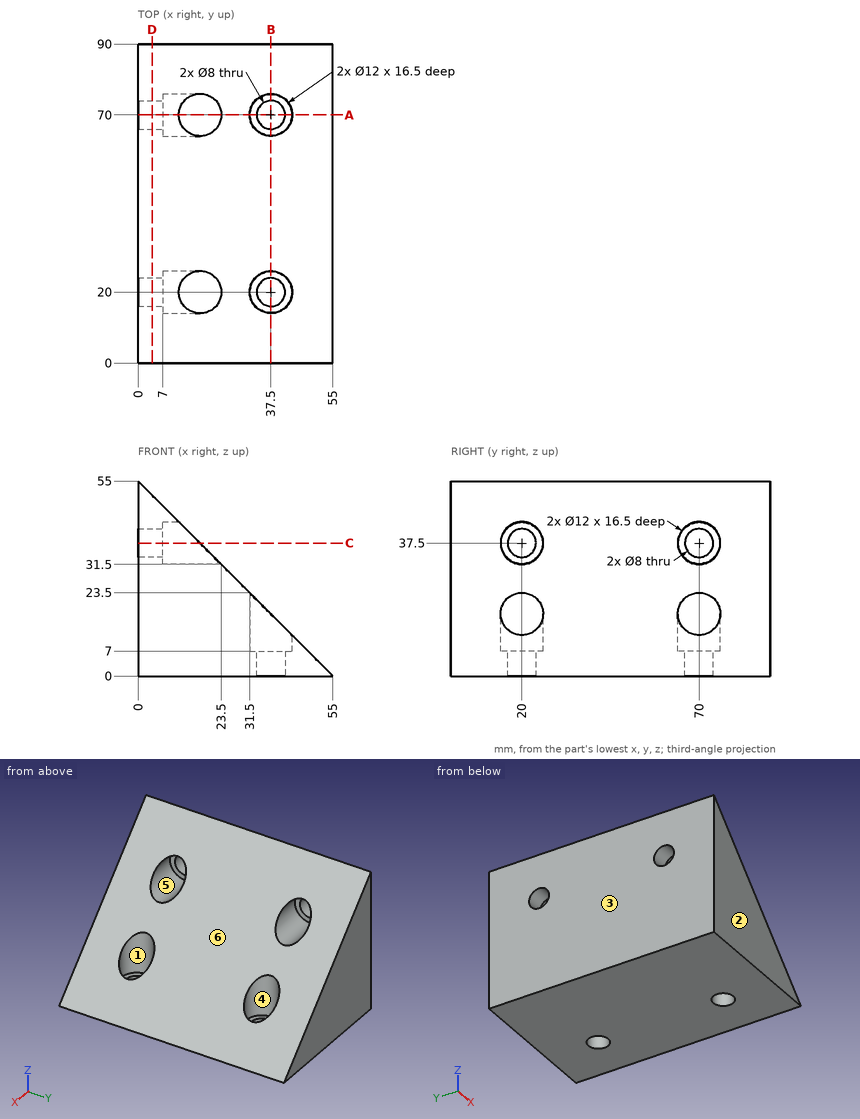
Drawing for the job (mm, zero at the part's lowest x, y, z). A direction names the side the tool comes from. Round coordinates to 2 decimals unless told otherwise and drop trailing zeros. Write each loop counter-clockwise with the first axis right and the second up, starting at its lowest first coordinate (ties: lowest second). Pieces come first, ordered by that corner, then holes. Notation, with made-up numbers: M 20.25,47 L 69.25,47 A21 cw 69.25,86 Z; hole C 9,54 d2. An arc over 180 degrees is marked long. Answer as a JSON object with one key per item and string values. Group by question number.
(1) Cut at B-B (x = 37.5). Give the cut face in (y, z), and give its area (3 significant figures).
(2) Flat gauge pins, fed straight in: pin 1 (13 mm diameter, centred on x = 35.5, y = 19.5, fed in from +Z); pin 2 (10.5 mm diameter, centred on y = 20, z = 37.5, fed in from +X); pin 3 (3.5 mm diameter, centred on x = 35, y = 69, fed in from +Z). Where does each tip first touch, or does it go through?
(3) Mould opens along X. For the marked faces 1, 2, 3 and 4 say: pulls with the +X half, pulls with the -X half, needs draft (parallel to the pull), parting line crosses it, or undercut.
(4) Which spindle directions (+Z, -Z, +X, -X, +Y, -Y) get a long thin tool onto all of the face, cutting with end or side? Do the marked faces 5 and 6. Say none if no direction does.
(5) Cut at D-D (x = 4). Give the cut face in (y, z), and give its area (3 significant figures).
(6) Cut at C-C (z = 37.5). Give the cut face in (x, y).
(7) Drill centre lines: L1, parallel to Y at x = 37, z = 13; L2, parallel to Y at x = 37.5, z = 3.5; L3, parallel to Z at x = 9.5, y = 73.5. Where is each one in solid material? Low to high.
(8) Cut at A-A (y = 70). Give the cut face in (x, z).
Responses:
{
 "1": {"outline": "M 0,0 L 16,0 L 16,7 L 14,7 L 14,17.5 L 0,17.5 Z; M 24,0 L 66,0 L 66,7 L 64,7 L 64,17.5 L 26,17.5 L 26,7 L 24,7 Z; M 74,0 L 90,0 L 90,17.5 L 76,17.5 L 76,7 L 74,7 Z", "area": "1,210 mm2"},
 "2": {"pin 1": "stops at z = 26", "pin 2": "stops at x = 7", "pin 3": "stops at z = 7"},
 "3": {"face 1": "undercut", "face 2": "needs draft", "face 3": "pulls with the -X half", "face 4": "undercut"},
 "4": {"face 5": "+X", "face 6": "+Z, +X, +Y, -Y"},
 "5": {"outline": "M 0,0 L 90,0 L 90,51 L 0,51 Z; hole C 20,37.5 d8; hole C 70,37.5 d8", "area": "4,490 mm2"},
 "6": {"outline": "M 0,0 L 17.5,0 L 17.5,14 L 7,14 L 7,16 L 0,16 Z; M 0,24 L 7,24 L 7,26 L 17.5,26 L 17.5,64 L 7,64 L 7,66 L 0,66 Z; M 0,74 L 7,74 L 7,76 L 17.5,76 L 17.5,90 L 0,90 Z"},
 "7": {"L1": "y = 0 to 14.02, 25.98 to 64.02, 75.98 to 90", "L2": "y = 0 to 16, 24 to 66, 74 to 90", "L3": "z = 0 to 32.63, 42.37 to 45.5"},
 "8": {"outline": "M 0,0 L 33.5,0 L 33.5,7 L 31.5,7 L 31.5,23.5 L 23.5,31.5 L 7,31.5 L 7,33.5 L 0,33.5 Z; M 0,41.5 L 7,41.5 L 7,43.5 L 11.5,43.5 L 0,55 Z; M 41.5,0 L 55,0 L 43.5,11.5 L 43.5,7 L 41.5,7 Z"}
}
